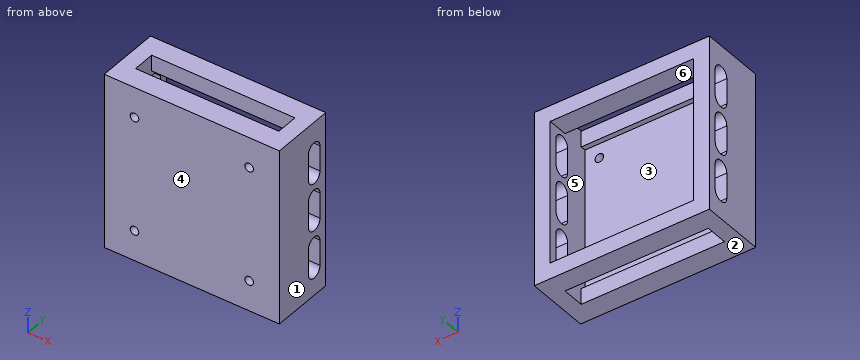
```python
from build123d import *

# Parameters (mm, degrees)
SKETCH1_W           = 45
SKETCH1_H           = 45
SKETCH1_R           = 1.35
BOSS_EXTRUDE1_DEPTH = 5
SKETCH2_W           = 55
SKETCH2_H           = 55
SKETCH2_W_2         = 45
SKETCH2_H_2         = 45
BOSS_EXTRUDE2_DEPTH = 20
SKETCH3_W           = 45
SKETCH3_H           = 6.969851319
CUT_EXTRUDE1_DEPTH  = 65.662585782
CUT_EXTRUDE2_DEPTH  = 65.662585782
CUT_EXTRUDE3_DEPTH  = 67.801946079


with BuildPart() as part:
    # Sketch1 → Boss-Extrude1 (new body)
    with BuildSketch(Plane(origin=(0, 0, 0), x_dir=(1, 0, 0), z_dir=(0, 1, 0))):
        Rectangle(SKETCH1_W, SKETCH1_H)
        with Locations(Location((-18, 18, 0), (0, 0, 270))):
            Circle(SKETCH1_R, mode=Mode.SUBTRACT)
        with Locations(Location((18, 18, 0), (0, 0, 270))):
            Circle(SKETCH1_R, mode=Mode.SUBTRACT)
        with Locations(Location((18, -18, 0), (0, 0, 270))):
            Circle(SKETCH1_R, mode=Mode.SUBTRACT)
        with Locations(Location((-18, -18, 0), (0, 0, 270))):
            Circle(SKETCH1_R, mode=Mode.SUBTRACT)
    extrude(amount=BOSS_EXTRUDE1_DEPTH)

    # Sketch2 → Boss-Extrude2 (add)
    with BuildSketch(Plane(origin=(0, 0, 0), x_dir=(1, 0, 0), z_dir=(0, 1, 0))):
        Rectangle(SKETCH2_W, SKETCH2_H)
        Rectangle(SKETCH2_W_2, SKETCH2_H_2, mode=Mode.SUBTRACT)
    extrude(amount=BOSS_EXTRUDE2_DEPTH)

    # Sketch3 → Cut-Extrude1 (cut, through all)
    with BuildSketch(Plane(origin=(0, 0, -27.5), x_dir=(-1, 0, 0), z_dir=(0, 0, -1))):
        with Locations((0, 10.115904606)):
            Rectangle(SKETCH3_W, SKETCH3_H)
    extrude(amount=-CUT_EXTRUDE1_DEPTH, mode=Mode.SUBTRACT)

    # Sketch4 → Cut-Extrude2 (cut, through all)
    with BuildSketch(Plane.ZY.offset(27.5)):
        with BuildLine():
            Line((-11.5, 12.5), (-19.5, 12.5))
            ThreePointArc((-19.5, 12.5), (-22, 15), (-19.5, 17.5))
            Line((-19.5, 17.5), (-11.5, 17.5))
            ThreePointArc((-11.5, 17.5), (-9, 15), (-11.5, 12.5))
        make_face()
        with BuildLine():
            Line((3.5, 17.5), (-4.5, 17.5))
            ThreePointArc((-4.5, 17.5), (-7, 15), (-4.5, 12.5))
            Line((-4.5, 12.5), (3.5, 12.5))
            ThreePointArc((3.5, 12.5), (6, 15), (3.5, 17.5))
        make_face()
        with BuildLine():
            Line((18.5, 17.5), (10.5, 17.5))
            ThreePointArc((10.5, 17.5), (8, 15), (10.5, 12.5))
            Line((10.5, 12.5), (18.5, 12.5))
            ThreePointArc((18.5, 12.5), (21, 15), (18.5, 17.5))
        make_face()
    extrude(amount=-CUT_EXTRUDE2_DEPTH, mode=Mode.SUBTRACT)

    # Sketch5 → Cut-Extrude3 (cut, through all)
    with BuildSketch(Plane(origin=(0, 0, -30), x_dir=(-1, 0, 0), z_dir=(0, 0, -1))):
        with BuildLine():
            Line((-7.5, 33), (7.5, 33))
            ThreePointArc((7.5, 33), (10.5, 30), (7.5, 27))
            Line((7.5, 27), (-7.5, 27))
            ThreePointArc((-7.5, 27), (-10.5, 30), (-7.5, 33))
        make_face()
    extrude(amount=-CUT_EXTRUDE3_DEPTH, mode=Mode.SUBTRACT)


solid = part.part
```
The listing builds one solid part. Answer for the finished solid, in the listing's coordinates (mm). Face numbers are marked on the shaded views. A direction names the side the tool comes from. Round coordinates to 2 decimals unless told otherwise and drop trailing zeros. Loops run counter-clockwise (first coordinate to the right, second up) from the corner with the lowest first, then second, coordinate; pieces in that order, holes last. Notation, with made-up numbers: (-26.5, 43) - (-22.5, 43) arc R12 cw to (-22.5, 53) - close; hole circle Ø10 at (14, -29.75). An arc over 180 degrees is marked (long way). Return JSON: item names as keys, results as strings. Group by question number.
1. The part is cut by section D-D on y = 15. State how many separate pieces and enclosed holes the cut face has, then the cut area to 3 significant figures.
2. Which of the six approach directions +Z, -Z, +X, -X, +Y, -Y give full straight-line access (tool end or side, diameter ignored) to the marked faces 4, 5 and 6?
3. The part is cut by section B-B on x = -18. Determine the outline of the cut face in (y, z).
4. Consider probe 1 along X at (y, z) = (3, -18); probe 2 along Z at (x, y) = (-21.5, 15.75); probe 3 along Y at (x, z) = (-24, 14). Determine where each line is inside the solid, lowest interval first.
5. This flat-tipped pin is pushed along its axis until it touches: P1, Ø3.5, axis at x = -18, z = -18, coming from the +Y side. Where does it stop, or does it pass through?
6. The mould has two halves that part along X. Classify the marked faces 1, 2 and 3: pulls with the +X half, pulls with the -X half, needs draft (parallel to the pull), parting line crosses it, or undercut.
7. The part is cut by section C-C on z = 2.5. Determine the outline of the cut face in (x, y), then the cut area to 3 significant figures.
8. The part is cut by section A-A on y = 9.25. Determine the outline of the cut face in (x, z), then the cut area to 3 significant figures.
Resolved:
{
 "1": {"separate pieces": "6", "enclosed holes": "0", "area": "610 mm²"},
 "2": {"face 4": "+Z, -Z, +X, -X, -Y", "face 5": "none", "face 6": "+Y"},
 "3": {"outline": "(0, -27.5) - (6.63, -27.5) - (6.63, -22.5) - (5, -22.5) - (5, -19.35) - (0, -19.35) - close; (0, -16.65) - (5, -16.65) - (5, 16.65) - (0, 16.65) - close; (0, 19.35) - (5, 19.35) - (5, 22.5) - (6.63, 22.5) - (6.63, 27.5) - (0, 27.5) - close; (13.6, -27.5) - (20, -27.5) - (20, -22.5) - (13.6, -22.5) - close; (13.6, 22.5) - (20, 22.5) - (20, 27.5) - (13.6, 27.5) - close"},
 "4": {"probe 1": "x = -27.5 to -19.35, -16.65 to 16.65, 19.35 to 27.5", "probe 2": "z = -27.5 to -22.5, 22.5 to 27.5", "probe 3": "y = 0 to 12.5, 17.5 to 20"},
 "5": {"P1": "stops at y = 5"},
 "6": {"face 1": "pulls with the +X half", "face 2": "needs draft", "face 3": "undercut"},
 "7": {"outline": "(-27.5, 0) - (27.5, 0) - (27.5, 12.5) - (22.5, 12.5) - (22.5, 5) - (-22.5, 5) - (-22.5, 12.5) - (-27.5, 12.5) - close; (-27.5, 17.5) - (-22.5, 17.5) - (-22.5, 20) - (-27.5, 20) - close; (22.5, 17.5) - (27.5, 17.5) - (27.5, 20) - (22.5, 20) - close", "area": "375 mm²"},
 "8": {"outline": "(-27.5, -27.5) - (-22.5, -27.5) - (-22.5, 27.5) - (-27.5, 27.5) - close; (22.5, -27.5) - (27.5, -27.5) - (27.5, 27.5) - (22.5, 27.5) - close", "area": "550 mm²"}
}
